Autodesk Inventor part; units mm, degrees
ref_plane "YZ Plane" through (0, 0, 0) normal (1, 0, 0) x (0, 1, 0)
ref_plane "XZ Plane" through (0, 0, 0) normal (0, 1, 0) x (-1, 0, 0)
ref_plane "XY Plane" through (0, 0, 0) normal (0, 0, 1) x (1, 0, 0)
sketch "Sketch2" plane through (0, 0, 0) normal (0, 0, 1) x (1, 0, 0)
  line L0 (-6.5, -6.5) -> (6.5, -6.5)
  line L1 (6.5, -6.5) -> (6.5, 6.5)
  line L2 (6.5, 6.5) -> (-6.5, 6.5)
  line L3 (-6.5, 6.5) -> (-6.5, -6.5)
  line L4 (-6.5, -6.5) -> (6.5, 6.5) construction
  line L5 (6.5, -6.5) -> (-6.5, 6.5) construction
  line L6 (-5.25, -5.25) -> (5.25, -5.25)
  line L7 (5.25, -5.25) -> (5.25, 5.25)
  line L8 (5.25, 5.25) -> (-5.25, 5.25)
  line L9 (-5.25, 5.25) -> (-5.25, -5.25)
  line L10 (-5.25, -5.25) -> (5.25, 5.25) construction
  line L11 (5.25, -5.25) -> (-5.25, 5.25) construction
  line L12 (-5.75, 5.75) -> (5.75, 5.75)
  line L13 (5.75, 5.75) -> (5.75, -5.75)
  line L14 (5.75, -5.75) -> (-5.75, -5.75)
  line L15 (-5.75, -5.75) -> (-5.75, 5.75)
  line L16 (-3.5, -3.5) -> (3.5, -3.5)
  line L17 (3.5, -3.5) -> (3.5, 3.5)
  line L18 (3.5, 3.5) -> (-3.5, 3.5)
  line L19 (-3.5, 3.5) -> (-3.5, -3.5)
  line L20 (-3.5, -3.5) -> (3.5, 3.5) construction
  line L21 (3.5, -3.5) -> (-3.5, 3.5) construction
  point P0 (0, 0)
  dimension "d0" = 13
  dimension "d1" = 13
  dimension "d2" = 10.5
  dimension "d3" = 10.5
  dimension "d4" = 0.5
  dimension "d5" = 7
  dimension "d6" = 7
extrude "Extrusion1" add sketch "Sketch2" along normal blind 3 contours L3 L2 L1 L0
extrude "Extrusion2" add sketch "Sketch2" along normal blind 1 contours L9 L8 L7 L6 | L12 L13 L14 L15 | L19 L18 L17 L16
extrude "Extrusion3" cut sketch "Sketch2" along normal blind 1 contours L19 L18 L17 L16
fillet "Fillet1" radius 2 4 edges at (-3.5, 3.5, 0.5) (-3.5, -3.5, 0.5) (3.5, 3.5, 0.5) (3.5, -3.5, 0.5)
chamfer "Chamfer1" distance 1 angle 45 8 edges at (0, 3.5, 0) (-2.9142, 2.9142, 0) (-3.5, 0, 0) (-2.9142, -2.9142, 0) (0, -3.5, 0) (2.9142, -2.9142, 0) (3.5, 0, 0) (2.9142, 2.9142, 0)
sketch "Sketch3" plane through (0, 0, 3) normal (0, 0, 1) x (1, 0, 0)
  line L0 (5.75, -5.75) -> (-5.75, -5.75)
  line L1 (-6.5, -6.5) -> (6.5, -6.5)
  line L2 (-5.75, -5.75) -> (5.75, -5.75)
  line L3 (5.75, -5.75) -> (5.75, -6.5)
  line L4 (5.75, -6.5) -> (-5.75, -6.5)
  line L5 (-5.75, -6.5) -> (-5.75, -5.75)
  point P0 (0, 0)
  dimension "d17" = 11.5
extrude "Extrusion4" cut sketch "Sketch3" against normal blind 1
properties part number "Optical module_lid" material "PET Plastic"
Geometry: final body of the model. Coordinates: model frame, mm. A direction names the side the tool comes from. Coordinates: 2 decimals unless noted, no trailing zeros. Order: outer loops, then holes, each group sorted by start corner. A loop starts at its lowest first (then second) coordinate and runs counter-clockwise, first axis right, second up. Notation, with made-up numbers: M -26.5,52.5 L -9.5,52.5 A13 cw -9.5,66.5 Z; hole C 80.5,73.25 d8. An arc over 180 degrees is marked long. Answer in a Markdown table with one row per item. Add a question column.
Q1. Mould query, pull axis X, two halves, no side actions, for faces 4 (the conical face through (-3.18, -3.21, 0.6)), 5 (the flat face through (6.5, 0, 1)), 6 (the flat face through (-1, 6, 3)). Classes: released by +X, released by -X, zero draft, split by the parting line, or undercut.
Q2. Contact query for flat-ended pins moving along their axis: P1, Ø0.6, axis at x = -0.5, y = -6.5, coming from the +Z side; P2, Ø6, axis at x = 2.5, y = 0.5, coming from the +Z side. Output: stop coordinate, or through.
Q3. Section query D-D on x = 4.75. Return the cut outline in (y, z), and give its area (4 significant figures).
Q4. Section query A-A on z = 1.6. Return the cut outline in (x, y), and give its area (4 significant figures).
Q5. Reachability of faces 1 (the flat face through (4, 0, 0.5)), 2 (the flat face through (0, 6.5, 1)), 3 (the flat face through (-5.75, 0, 2)) from +Z, -Z, +X, -X, +Y, -Y: full face, straight path, thin tool, end or side. Return the list, or none.
Q6. Section query C-C on y = -5. Return the cut outline in (x, z), and give its area (3 significant figures).
Q7. Line query: L1, parallel to X at y = -5.5, z = 1.75; L2, parallel to Z at x = -5.5, y = 1.25. Output: solid intervals per line, ascending.
Completed:
| question | item | result |
|---|---|---|
| 1 | face 4 | undercut |
| 1 | face 5 | released by +X |
| 1 | face 6 | zero draft |
| 2 | P1 | stops at z = 2 |
| 2 | P2 | stops at z = 1 |
| 3 | outline | M -6.5,0 L 6.5,0 L 6.5,3 L 5.75,3 L 5.75,1 L -5.75,1 L -5.75,2 L -6.5,2 Z |
| 3 | area | 15.25 mm2 |
| 4 | outline | M -6.5,-6.5 L 6.5,-6.5 L 6.5,6.5 L -6.5,6.5 Z; hole M -5.75,-5.75 L 5.75,-5.75 L 5.75,5.75 L -5.75,5.75 Z |
| 4 | area | 36.75 mm2 |
| 5 | face 1 | -Z |
| 5 | face 2 | +Z, -Z, +X, -X, +Y |
| 5 | face 3 | +Z |
| 6 | outline | M -6.5,0 L 6.5,0 L 6.5,3 L 5.75,3 L 5.75,1 L -5.75,1 L -5.75,3 L -6.5,3 Z |
| 6 | area | 16.0 mm2 |
| 7 | L1 | x = -6.5 to -5.75, 5.75 to 6.5 |
| 7 | L2 | z = 0 to 1 |
